The listing builds one solid part. Answer for the finished solid, in the listing's coordinates (mm). Face numbers are marked on the shaded views. A direction names the side the tool comes from. Coordinates: 2 decimals unless noted, no trailing zeros. Order: outer loops, then holes, each group sorted by start corner. A loop starts at its lowest first (then second) coordinate and runs counter-clockwise, first axis right, second up. Notation, with made-up numbers: (-21.5, 89.25) - (16.5, 89.25) arc R16 ccw to (16.5, 101.25) - close; hole circle Ø8 at (-25, 84). An arc over 180 degrees is marked (long way). One line per item, written item: value. Start each with the question number.
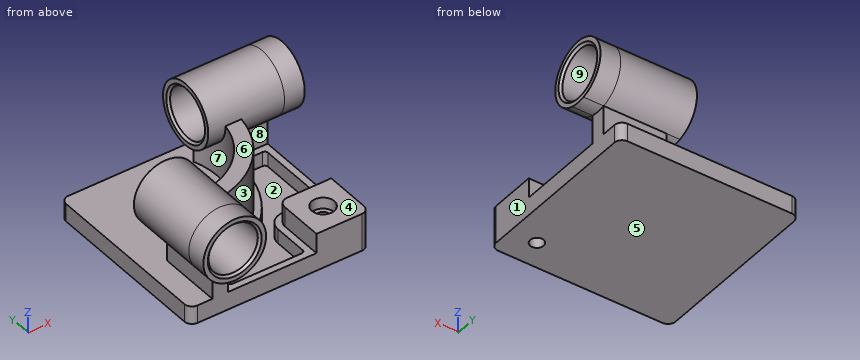
```python
from build123d import *

# Parameters (mm, degrees)
F0_W            = 101.6
F0_H            = 101.6
F1_DEPTH        = 10.16
F3_DEPTH        = 33.528
F5_DEPTH        = 11.43
F5_DEPTH_BACK   = 43.18
F7_DEPTH        = 11.43
F7_DEPTH_BACK   = 43.18
F8_W            = 29.972
F8_H            = 29.972
F9_DEPTH        = 11.176
F10_R           = 5.08
F12_DEPTH       = 8.128
F14_D           = 7.62
F14_CBORE_D     = 12.7
F14_CBORE_DEPTH = 6.35
F15_R           = 1.778
F16_R           = 13.97
F17_DEPTH       = 86.868
F18_R           = 13.97
F19_DEPTH       = 107.696
F20_SIZE        = 1.27
F21_R           = 4.318


with BuildPart() as f1:
    # F0 (on Top) → F1 (new body)
    with BuildSketch(Plane.XY):
        Rectangle(F0_W, F0_H)
    extrude(amount=F1_DEPTH)

    # F2 (on face) → F3 (join)
    with BuildSketch(Plane.XY.offset(10.16)):
        with BuildLine():
            Line((-38.1, -15.24), (-38.1, -50.8))
            Line((-38.1, -50.8), (-29.2099993676, -50.8))
            Line((-29.2099993676, -50.8), (-29.2099993676, -26.5417011038))
            ThreePointArc((-29.2099993676, -26.5417011038), (12.2116619609, -12.2116619609), (26.5417011038, 29.2099993676))
            Line((26.5417011038, 29.2099993676), (50.8, 29.2099993676))
            Line((50.8, 29.2099993676), (50.8, 38.1))
            Line((50.8, 38.1), (15.24, 38.1))
            ThreePointArc((15.24, 38.1), (5.9254822289, -5.9254822289), (-38.1, -15.24))
        make_face()
    extrude(amount=F3_DEPTH)

    # F4 (on face) → F5 (join, two sides)
    with BuildSketch(Plane.XZ.offset(50.8)) as f5_sk:
        with BuildLine():
            ThreePointArc((-29.2099993676, 26.4725891078), (-19.5986753844, 32.8000182224), (-15.8749996838, 43.688))
            ThreePointArc((-15.8749996838, 43.688), (-44.5429814614, 57.7443242994), (-38.1, 26.4725891078))
            Line((-38.1, 26.4725891078), (-38.1, 43.688))
            Line((-38.1, 43.688), (-29.2099993676, 43.688))
            Line((-29.2099993676, 43.688), (-29.2099993676, 26.4725891078))
        make_face()
        with BuildLine():
            Line((-38.1, 43.688), (-38.1, 26.4725891078))
            ThreePointArc((-38.1, 26.4725891078), (-33.6549996838, 25.908), (-29.2099993676, 26.4725891078))
            Line((-29.2099993676, 26.4725891078), (-29.2099993676, 43.688))
            Line((-29.2099993676, 43.688), (-38.1, 43.688))
        make_face()
    extrude(amount=F5_DEPTH)
    extrude(f5_sk.sketch, amount=-F5_DEPTH_BACK)

    # F6 (on face) → F7 (join, two sides)
    with BuildSketch(Plane.YZ.offset(50.8)) as f7_sk:
        with BuildLine():
            ThreePointArc((38.1, 26.4725891078), (47.7113239832, 32.8000182224), (51.4349996838, 43.688))
            ThreePointArc((51.4349996838, 43.688), (22.7670179062, 57.7443242994), (29.2099993676, 26.4725891078))
            Line((29.2099993676, 26.4725891078), (29.2099993676, 43.688))
            Line((29.2099993676, 43.688), (38.1, 43.688))
            Line((38.1, 43.688), (38.1, 26.4725891078))
        make_face()
        with BuildLine():
            Line((29.2099993676, 43.688), (29.2099993676, 26.4725891078))
            ThreePointArc((29.2099993676, 26.4725891078), (33.6549996838, 25.908), (38.1, 26.4725891078))
            Line((38.1, 26.4725891078), (38.1, 43.688))
            Line((38.1, 43.688), (29.2099993676, 43.688))
        make_face()
    extrude(amount=F7_DEPTH)
    extrude(f7_sk.sketch, amount=-F7_DEPTH_BACK)

    # F8 (on face) → F9 (join)
    with BuildSketch(Plane.XY.offset(10.16)):
        with Locations((35.814, -35.814)):
            Rectangle(F8_W, F8_H)
    extrude(amount=F9_DEPTH)

    # F10
    f10_edges = [f1.edges().sort_by_distance(p)[0] for p in [
        (20.828, -20.828, 15.748),
    ]]
    fillet(f10_edges, radius=F10_R)

    # F11 (on face) → F12 (cut)
    with BuildSketch(Plane.XY.offset(10.16)):
        with BuildLine():
            ThreePointArc((30.6647931111, 25.3999990791), (14.9057390012, -14.9057390012), (-25.3999990791, -30.6647931111))
            Line((-25.3999990791, -30.6647931111), (-25.3999990791, -46.9899997115))
            Line((-25.3999990791, -46.9899997115), (17.0179997115, -46.9899997115))
            Line((17.0179997115, -46.9899997115), (17.0179997115, -25.908))
            ThreePointArc((17.0179997115, -25.908), (19.6218205113, -19.6218205113), (25.908, -17.0179997115))
            Line((25.908, -17.0179997115), (46.9899997115, -17.0179997115))
            Line((46.9899997115, -17.0179997115), (46.9899997115, 25.3999990791))
            Line((46.9899997115, 25.3999990791), (30.6647931111, 25.3999990791))
        make_face()
    extrude(amount=-F12_DEPTH, mode=Mode.SUBTRACT)

    # F14 (through all)
    with Locations(Plane.XY.offset(21.336)):
        with Locations((35.56, -35.56)):
            CounterBoreHole(F14_D / 2, F14_CBORE_D / 2, F14_CBORE_DEPTH)

    # F15
    f15_edges = [f1.edges().sort_by_distance(p)[0] for p in [
        (-25.399999, -46.99, 6.096),
        (-25.399999, -30.664793, 6.096),
        (30.664793, 25.399999, 6.096),
        (46.99, 25.399999, 6.096),
        (46.99, -17.018, 6.096),
        (17.018, -46.99, 6.096),
    ]]
    fillet(f15_edges, radius=F15_R)

    # F16 (on face) → F17 (cut)
    with BuildSketch(Plane.XZ.offset(62.23)):
        with Locations((-33.6549996838, 43.688)):
            Circle(F16_R)
    extrude(amount=-F17_DEPTH, mode=Mode.SUBTRACT)

    # F18 (on face) → F19 (cut)
    with BuildSketch(Plane.YZ.offset(62.23)):
        with Locations((33.6549996838, 43.688)):
            Circle(F18_R)
    extrude(amount=-F19_DEPTH, mode=Mode.SUBTRACT)

    # F20
    f20_edges = [f1.edges().sort_by_distance(p)[0] for p in [
        (62.23, 19.685, 43.688),
        (-47.625, -62.23, 43.688),
        (7.62, 19.685, 43.688),
        (-47.625, -7.62, 43.688),
    ]]
    chamfer(f20_edges, length=F20_SIZE)

    # F21
    f21_edges = [f1.edges().sort_by_distance(p)[0] for p in [
        (50.8, -50.8, 10.668),
        (50.8, 50.8, 5.08),
        (-50.8, 50.8, 5.08),
        (-50.8, -50.8, 5.08),
    ]]
    fillet(f21_edges, radius=F21_R)


solid = f1.part
```
(1) For a pull along Z with two mould halves and no side action, classify the marked faces 1, 2, 3 and 4 as pulls with the +Z half, pulls with the -Z half, needs draft (parallel to the pull), parting line crosses it, or undercut.
(2) The part is cut by section C-C on y = -35.56. Determine the outline of the cut face in (x, z) (3 decimals), plus the area to 3 significant figures.
(3) The part is cut by section A-A on x = 35.56. Determine the outline of the cut face in (y, z) (3 decimals).
(4) The part is cut by section D-D on x = -5. Determine the outline of the cut face in (y, z).
(5) Consider probe 1 along X at (y, z) = (-35, 16); probe 2 along Y at (x, z) = (35, 17); probe 3 along Y at (x, z) = (35.5, 14). Determine where each line is inside the solid, lowest interval first.
(6) Flat-ended cylindrical pins translate along their axes: pin 1 Ø8 at (y, z) = (-35.5, 17.5) entering from +X; pin 2 Ø3 at (x, z) = (15.5, 4) entering from +Y; pin 3 Ø18 at (x, z) = (36, 22) entering from -Y; pin 4 Ø25 at (x, z) = (-33.655, 43.688) entering from -Y. Find the tip coordinate at first contact, or state that the pin passes through.
(7) The part is cut by section B-B on z = 12. Determine the outline of the cut face in (x, y).
(8) For the marked faces 5, 6, 7, 8 and 9, determine the directions among +Z, -Z, +X, -X, +Y, -Y from which every point of the face is accessible in a straight line to the end or side of a thin tool.
Completed:
1. face 1: needs draft
1. face 2: undercut
1. face 3: undercut
1. face 4: pulls with the +Z half
2. outline: (-50.8, 0) - (31.75, 0) - (31.75, 14.986) - (29.21, 14.986) - (29.21, 21.336) - (20.828, 21.336) - (20.828, 10.16) - (17.018, 10.16) - (17.018, 2.032) - (-25.4, 2.032) - (-25.4, 10.16) - (-29.21, 10.16) - (-29.21, 26.473) arc R17.78 ccw (long way) to (-38.1, 26.473) - (-38.1, 10.16) - (-50.8, 10.16) - close; (39.37, 0) - (50.8, 0) - (50.8, 21.336) - (41.91, 21.336) - (41.91, 14.986) - (39.37, 14.986) - close; hole circle Ø27.94 at (-33.655, 43.688)
2. area: 1,350 mm2
3. outline: (-50.8, 0) - (-39.37, 0) - (-39.37, 14.986) - (-41.91, 14.986) - (-41.91, 21.336) - (-50.8, 21.336) - close; (-31.75, 0) - (50.8, 0) - (50.8, 10.16) - (38.1, 10.16) - (38.1, 26.473) arc R17.78 ccw (long way) to (29.21, 26.473) - (29.21, 10.16) - (25.4, 10.16) - (25.4, 2.032) - (-17.018, 2.032) - (-17.018, 10.16) - (-20.828, 10.16) - (-20.828, 21.336) - (-29.21, 21.336) - (-29.21, 14.986) - (-31.75, 14.986) - close; hole circle Ø27.94 at (33.655, 43.688)
4. outline: (-50.8, 0) - (50.8, 0) - (50.8, 10.16) - (-13.75, 10.16) - (-13.75, 43.69) - (-23.46, 43.69) - (-23.46, 10.16) - (-27.53, 10.16) - (-27.53, 2.03) - (-46.99, 2.03) - (-46.99, 10.16) - (-50.8, 10.16) - close
5. probe 1: x = -38.1 to -29.21, 20.83 to 29.23, 41.89 to 50.8
5. probe 2: y = -50.8 to -41.89, -29.23 to -20.83, 29.21 to 38.1
5. probe 3: y = -50.8 to -39.37, -31.75 to -20.83, 29.21 to 38.1
6. pin 1: stops at x = 50.8
6. pin 2: stops at y = 50.8
6. pin 3: stops at y = -50.8
6. pin 4: passes through
7. outline: (-38.1, -50.8) - (-29.21, -50.8) - (-29.21, -26.54) arc R50.14 ccw to (26.54, 29.21) - (50.8, 29.21) - (50.8, 38.1) - (15.24, 38.1) arc R41.25 cw to (-38.1, -15.24) - close; (20.83, -50.8) - (46.48, -50.8) arc R4.32 ccw to (50.8, -46.48) - (50.8, -20.83) - (25.91, -20.83) arc R5.08 ccw to (20.83, -25.91) - close; hole circle Ø7.62 at (35.56, -35.56)
8. face 5: -Z, +X, -X, +Y, -Y
8. face 6: +Z, +X, -Y
8. face 7: none
8. face 8: +X
8. face 9: +X, -X
